from build123d import *

# Parameters (mm, degrees)
SKETCH1_R                  = 17
BOSS_EXTRUDE1_DEPTH        = 8
SKETCH9_W                  = 6
SKETCH9_H                  = 13.19
CUT_EXTRUDE1_DEPTH         = 26.337718919
SKETCH10_R                 = 2.5
CUT_EXTRUDE2_DEPTH         = 6.35
FILLET2_R                  = 1
CIRPATTERN2_COUNT          = 3
FILLET2_OF_CIRPATTERN2_R   = 1
SKETCH12_R                 = 20
CUT_EXTRUDE3_DEPTH         = 10
F_2_2_2_2_DIAMETER_HOLE1_D = 2.2
FILLET3_R                  = 0.25


with BuildPart() as part:
    # Sketch1 → Boss-Extrude1 (new body)
    with BuildSketch(Plane(origin=(0, 0, 0), x_dir=(1, 0, 0), z_dir=(0, 1, 0))):
        with Locations(Location((0, 0, 0), (0, 0, 270))):
            Circle(SKETCH1_R)
    extrude(amount=BOSS_EXTRUDE1_DEPTH)

    # Sketch9 → Cut-Extrude1 (cut, through all)
    with BuildSketch(Plane(origin=(0, 8, 0), x_dir=(1, 0, 0), z_dir=(0, 1, 0))):
        with Locations((0, 10.405)):
            Rectangle(SKETCH9_W, SKETCH9_H)
    cut_extrude1 = extrude(amount=-CUT_EXTRUDE1_DEPTH, mode=Mode.SUBTRACT)

    # Sketch10 → Cut-Extrude2 (cut, symmetric)
    with BuildSketch(Plane(origin=(0, 0, 0), x_dir=(0, 0, -1), z_dir=(1, 0, 0))):
        with Locations((11.5, 4)):
            Circle(SKETCH10_R)
    cut_extrude2 = extrude(amount=CUT_EXTRUDE2_DEPTH, both=True, mode=Mode.SUBTRACT)

    # Fillet2
    fillet2_edges = [part.edges().sort_by_distance(p)[0] for p in [
        (-3, 4, -3.81),
        (3, 4, -3.81),
    ]]
    fillet(fillet2_edges, radius=FILLET2_R)

    # CirPattern2: Cut-Extrude1, Cut-Extrude2 ×3 about axis
    cirpattern2_axis = Axis((0, 0, 0), (0, 1, 0))
    add([cut_extrude1.rotate(cirpattern2_axis, i * 360 / CIRPATTERN2_COUNT) for i in range(1, CIRPATTERN2_COUNT)], mode=Mode.SUBTRACT)
    add([cut_extrude2.rotate(cirpattern2_axis, i * 360 / CIRPATTERN2_COUNT) for i in range(1, CIRPATTERN2_COUNT)], mode=Mode.SUBTRACT)

    # Fillet2 of CirPattern2
    fillet2_of_cirpattern2_edges = [part.edges().sort_by_distance(p)[0] for p in [
        (-1.799556788, 4, 4.503076211),
        (-4.799556788, 4, -0.693076211),
        (4.799556788, 4, -0.693076211),
        (1.799556788, 4, 4.503076211),
    ]]
    fillet(fillet2_of_cirpattern2_edges, radius=FILLET2_OF_CIRPATTERN2_R)

    # Sketch12 → Cut-Extrude3 (cut)
    with BuildSketch(Plane(origin=(0, 4, 0), x_dir=(1, 0, 0), z_dir=(0, 1, 0))):
        Circle(SKETCH12_R)
    extrude(amount=CUT_EXTRUDE3_DEPTH, mode=Mode.SUBTRACT)

    # 2.2 _2.2_ Diameter Hole1 (through all)
    with Locations(Plane.XZ):
        with Locations((-11.258330249, -6.5), (11.258330249, -6.5), (0, 13), (-7.361215932, -4.25), (7.361215932, -4.25), (0, 8.5)):
            Hole(F_2_2_2_2_DIAMETER_HOLE1_D / 2)

    # Fillet3
    fillet3_edges = [part.edges().sort_by_distance(p)[0] for p in [
        (-6.784292144, 1.5, 11.249261314),
        (-13.134292144, 1.5, 0.250738686),
        (13.134292144, 1.5, 0.250738686),
        (6.784292144, 1.5, 11.249261314),
        (-6.35, 1.5, -11.5),
        (6.35, 1.5, -11.5),
    ]]
    fillet(fillet3_edges, radius=FILLET3_R)


solid = part.part
Read the model definition and answer for the solid it produces. Units are mm, in the model's axes. A direction names the side the tool comes from. Coordinates: 2 decimals unless noted, no trailing zeros. Order: outer loops, then holes, each group sorted by start corner. A loop starts at its lowest first (then second) coordinate and runs counter-clockwise, first axis right, second up. Notation, with made-up numbers: M -39.75,18.25 L 7.25,18.25 A15 ccw 7.25,43.25 Z; hole C 38,47.25 d3. An arc over 180 degrees is marked long. Put each result on its own line as item: value. Start each with the question number.
Item 1: Section C-C, the plane z = -11.5 is taken. Determine the outline of the cut face in (x, y), plus the area to 3 significant figures.
Item 2: For faces 1 (the face through (4.6, 1.5, -11.4)), 2 (the face through (-4.9, 1.97, -0.29)), 3 (the face through (-3, 1, -11)), determine the directions among +Z, -Z, +X, -X, +Y, -Y from which every point of the face is accessible in a straight line to the end or side of a thin tool.
Item 3: The mould has two halves that part along Z. Classify faces 4 (the face through (2.715, 1.972, -4.111)), 5 (the face through (-6.55, 2.03, -3.51)), 6 (the face through (-14.618, 1.972, -8.679)): +Z half, -Z half, draft (parallel to the pull), parting line (faces both ways), or undercut.
Item 4: Given pin 1 Ø1.1 at (y, z) = (2.5, -12) entering from -X; pin 2 Ø1.5 at (x, y) = (-3, 1) entering from +Z; pin 3 Ø2 at (y, z) = (3, 11) entering from -X, each flat-ended and moving along its own axis, determine where each tip first touches the part or whether it passes through.
Item 5: Consider probe 1 along Z at (x, y) = (0, 0.9); probe 2 along X at (y, z) = (0.85, -4); probe 3 along X at (y, z) = (3.15, 3). Determine where each line is inside the solid, lowest interval first. Write a range as [from, to].
Item 6: Section A-A, the plane y = 1.1 is taken. Determine the outline of the cut face in (x, z), plus the area to 3 significant figures.
Item 7: Section B-B, the plane x = 0 is taken. Determine the outline of the cut face in (y, z).
Item 8: Section D-D, the plane z = -6.5 is taken. Determine the outline of the cut face in (x, y).
Computed:
1. outline: M -12.52,0 L -3,0 L -3,1.5 L -6.1,1.5 A0.25 cw -6.35,1.75 L -6.35,4 L -12.52,4 Z; M 3,0 L 12.52,0 L 12.52,4 L 6.35,4 L 6.35,1.75 A0.25 cw 6.1,1.5 L 3,1.5 Z
1. area: 59.4 mm2
2. face 1: +Y
2. face 2: +Y, -Y
2. face 3: -Z, +Y, -Y
3. face 4: -Z half
3. face 5: undercut
3. face 6: parting line
4. pin 1: stops at x = -12.57
4. pin 2: stops at z = 16.85
4. pin 3: stops at x = -12.99
5. probe 1: z = [-3.81, 7.4], [9.6, 11.9], [14.1, 17]
5. probe 2: x = [-16.52, -8.43], [-6.29, -2.59], [2.59, 6.29], [8.43, 16.52]
5. probe 3: x = [-16.73, -14.26], [-2.67, 2.67], [14.26, 16.73]
6. outline: M -15.99,5.77 A17 ccw -3,-16.73 L -3,-4.81 A1 cw -2,-3.81 L 2,-3.81 A1 cw 3,-4.81 L 3,-16.73 A17 ccw 15.99,5.77 L 5.67,-0.19 A1 cw 4.3,0.17 L 2.3,3.64 A1 cw 2.67,5 L 12.99,10.96 A17 ccw -12.99,10.96 L -2.67,5 A1 cw -2.3,3.64 L -4.3,0.17 A1 cw -5.67,-0.19 Z; hole C -11.26,-6.5 d2.2; hole C -7.36,-4.25 d2.2; hole C 0,8.5 d2.2; hole C 0,13 d2.2; hole C 7.36,-4.25 d2.2; hole C 11.26,-6.5 d2.2
6. area: 651 mm2
7. outline: M 0,-3.81 L 4,-3.81 L 4,7.4 L 0,7.4 Z; M 0,9.6 L 4,9.6 L 4,11.9 L 0,11.9 Z; M 0,14.1 L 4,14.1 L 4,17 L 0,17 Z
8. outline: M -15.71,0 L -12.36,0 L -12.36,4 L -15.71,4 Z; M -10.16,0 L -3,0 L -3,4 L -10.16,4 Z; M 3,0 L 10.16,0 L 10.16,4 L 3,4 Z; M 12.36,0 L 15.71,0 L 15.71,4 L 12.36,4 Z
